Read the model definition and answer for the solid it produces. Units are mm, in the model's axes. Face numbers are marked on the shaded views. A direction names the side the tool comes from. Give positions to 0.01 mm unless a question says otherwise; leave off trailing zeros. Order: outer loops, then holes, each group sorted by start corner. A loop starts at its lowest first (then second) coordinate and runs counter-clockwise, first axis right, second up. Notation, with made-up numbers: (62, -36.5) - (103, -36.5) arc R34 cw to (103, -5.5) - close; hole circle Ø10 at (89, 7.25). An arc over 180 degrees is marked (long way). Write each question's results on one line, items separated by ' | '. Start each with the question number.
Q1. Find section C-C on y = 19.75. Give the vertices of the cut face in (x, z).
Q2. Find the intervals of material crossed by line 1 along Y through (x, z) = (0.5, -6); line 2 along X through (y, z) = (18.5, 0); line 3 along X through (y, z) = (15, 2), in increasing order. Write a range as from..to.
Q3. A tool of negligible diameter and unlimited length cuts with its end or side. For the marked faces 1 and 2, from which of +Z, -Z, +X, -X, +Y, -Y can it reach the whole face along a straight path? Write none if from no direction.
Q4. Find section B-B on z = 0. Give the vertices of the cut face in (x, y).
Q5. Find section D-D on y = 8. Give the vertices of the cut face in (x, z), and give its area (3 significant figures).
Q6. Flat-ended cylindrical pins translate along their axes: P1, Ø3, axis at x = 0, z = 1.5, coming from the -Y side; P2, Ø8, axis at x = -1.5, y = 17.5, coming from the +Z side; P3, Ø5, axis at x = 4, y = 5.5, coming from the -Z side. Find the tip coordinate at first contact, or state that the pin passes through.
Q7. Find section A-A on x = 0. Give the vertices of the cut face in (y, z).
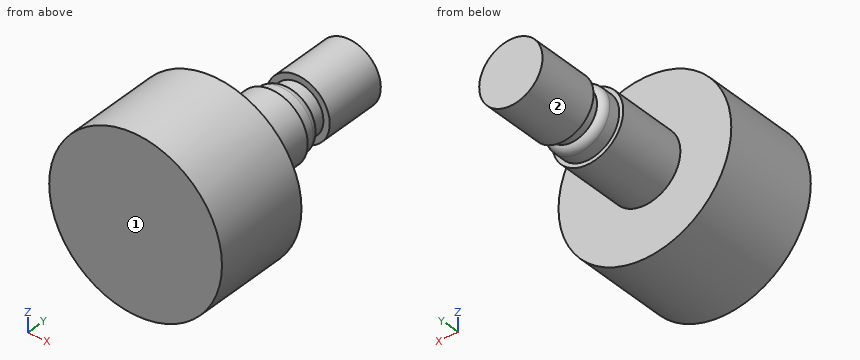
from build123d import *

# Parameters (mm, degrees)
SKETCH2_R           = 8.1915
BOSS_EXTRUDE1_DEPTH = 9.2583
SKETCH4_R           = 3.3655
BOSS_EXTRUDE3_DEPTH = 6.6548
SKETCH5_R           = 2.9845
BOSS_EXTRUDE4_DEPTH = 1.8669
FILLET1_R           = 0.762
SKETCH7_R           = 2.4003
BOSS_EXTRUDE5_DEPTH = 1.143
SKETCH8_R           = 3.00355
BOSS_EXTRUDE6_DEPTH = 5.9436


with BuildPart() as part:
    # Sketch2 → Boss-Extrude1 (new body)
    with BuildSketch(Plane(origin=(0, 0, 0), x_dir=(1, 0, 0), z_dir=(0, 1, 0))):
        with Locations(Location((0, 0, 0), (0, 0, 270))):
            Circle(SKETCH2_R)
    extrude(amount=BOSS_EXTRUDE1_DEPTH)

    # Sketch4 → Boss-Extrude3 (add)
    with BuildSketch(Plane(origin=(0, 9.2583, 0), x_dir=(1, 0, 0), z_dir=(0, 1, 0))):
        with Locations(Location((0, 0, 0), (0, 0, 270))):
            Circle(SKETCH4_R)
    extrude(amount=BOSS_EXTRUDE3_DEPTH)

    # Sketch5 → Boss-Extrude4 (add)
    with BuildSketch(Plane(origin=(0, 15.9131, 0), x_dir=(1, 0, 0), z_dir=(0, 1, 0))):
        with Locations(Location((0, 0, 0), (0, 0, 270))):
            Circle(SKETCH5_R)
    extrude(amount=BOSS_EXTRUDE4_DEPTH)

    # Fillet1
    fillet1_edges = [part.edges().sort_by_distance(p)[0] for p in [
        (0, 17.78, -2.9845),
    ]]
    fillet(fillet1_edges, radius=FILLET1_R)

    # Sketch7 → Boss-Extrude5 (add)
    with BuildSketch(Plane(origin=(0, 17.78, 0), x_dir=(1, 0, 0), z_dir=(0, 1, 0))):
        with Locations(Location((0, 0, 0), (0, 0, 270))):
            Circle(SKETCH7_R)
    extrude(amount=BOSS_EXTRUDE5_DEPTH)

    # Sketch8 → Boss-Extrude6 (add)
    with BuildSketch(Plane(origin=(0, 18.923, 0), x_dir=(1, 0, 0), z_dir=(0, 1, 0))):
        with Locations(Location((0, 0, 0), (0, 0, 270))):
            Circle(SKETCH8_R)
    extrude(amount=BOSS_EXTRUDE6_DEPTH)


solid = part.part
Working result:
1) outline: circle Ø6.01 at (0, 0)
2) line 1: 0..9.26 | line 2: -2.4..2.4 | line 3: -2.71..2.71
3) face 1: +Z, -Z, +X, -X, -Y | face 2: +Y
4) outline: (-8.19, 0) - (8.19, 0) - (8.19, 9.26) - (3.37, 9.26) - (3.37, 15.91) - (2.98, 15.91) - (2.98, 17.02) arc R0.76 ccw to (2.22, 17.78) - (2.4, 17.78) - (2.4, 18.92) - (3, 18.92) - (3, 24.87) - (-3, 24.87) - (-3, 18.92) - (-2.4, 18.92) - (-2.4, 17.78) - (-2.22, 17.78) arc R0.76 ccw to (-2.98, 17.02) - (-2.98, 15.91) - (-3.37, 15.91) - (-3.37, 9.26) - (-8.19, 9.26) - close
5) outline: circle Ø16.38 at (0, 0) | area: 211 mm²
6) P1: y = 0 | P2: z = 3.37 | P3: z = -8.05
7) outline: (0, -8.19) - (9.26, -8.19) - (9.26, -3.37) - (15.91, -3.37) - (15.91, -2.98) - (17.02, -2.98) arc R0.76 ccw to (17.78, -2.22) - (17.78, -2.4) - (18.92, -2.4) - (18.92, -3) - (24.87, -3) - (24.87, 3) - (18.92, 3) - (18.92, 2.4) - (17.78, 2.4) - (17.78, 2.22) arc R0.76 ccw to (17.02, 2.98) - (15.91, 2.98) - (15.91, 3.37) - (9.26, 3.37) - (9.26, 8.19) - (0, 8.19) - close
